from build123d import *

# Parameters (mm, degrees)
F0_W      = 30
F0_H      = 30
F1_DEPTH  = 20
F3_DEPTH  = 30.001
F7_W      = 5
F7_H      = 4
F8_DEPTH  = 3
F10_DEPTH = 1.5
F11_W     = 20
F11_H     = 12.5
F12_DEPTH = 9.9508743711
F13_W     = 30
F13_H     = 8
F14_DEPTH = 2
F15_R     = 1.25
F16_DEPTH = 5


with BuildPart() as f1:
    # F0 (on Front) → F1 (new body)
    with BuildSketch(Plane.XZ):
        with Locations((15, 15)):
            Rectangle(F0_W, F0_H)
    extrude(amount=F1_DEPTH)

    # F2 (on face) → F3 (cut, through all)
    with BuildSketch(Plane.XY.offset(30)):
        with BuildLine():
            Line((0, -20), (30, -20))
            ThreePointArc((30, -20), (15, -11.9498743711), (0, -20))
        make_face()
    extrude(amount=-F3_DEPTH, mode=Mode.SUBTRACT)

    # F7 (on offset) → F8 (cut)
    with BuildSketch(Plane.XZ.offset(12.9498743711)):
        with Locations((15, 15)):
            Rectangle(F7_W, F7_H)
    extrude(amount=-F8_DEPTH, mode=Mode.SUBTRACT)

    # F9 (on face) → F10 (cut)
    with BuildSketch(Plane.XY.offset(13)):
        with BuildLine():
            ThreePointArc((12.5, -12.1243309011), (15, -11.9498743711), (17.5, -12.1243309011))
            Line((17.5, -12.1243309011), (17.5, -9.9498743711))
            Line((17.5, -9.9498743711), (12.5, -9.9498743711))
            Line((12.5, -9.9498743711), (12.5, -12.1243309011))
        make_face()
    extrude(amount=-F10_DEPTH, mode=Mode.SUBTRACT)

    # F11 (on face) → F12 (cut, through all)
    with BuildSketch(Plane.XZ.offset(9.9498743711)):
        with Locations((15, 6.25)):
            Rectangle(F11_W, F11_H)
    extrude(amount=-F12_DEPTH, mode=Mode.SUBTRACT)

    # F13 (on face) → F14 (cut)
    with BuildSketch(Plane.XZ):
        with Locations((15, 15)):
            Rectangle(F13_W, F13_H)
    extrude(amount=F14_DEPTH, mode=Mode.SUBTRACT)

    # F15 (on face) → F16 (cut)
    with BuildSketch(Plane(origin=(0, 0, 12.5), x_dir=(1, 0, 0), z_dir=(0, 0, -1))):
        with Locations((18, 6.9498743711)):
            Circle(F15_R)
        with Locations((12, 6.9498743711)):
            Circle(F15_R)
    extrude(amount=-F16_DEPTH, mode=Mode.SUBTRACT)


solid = f1.part
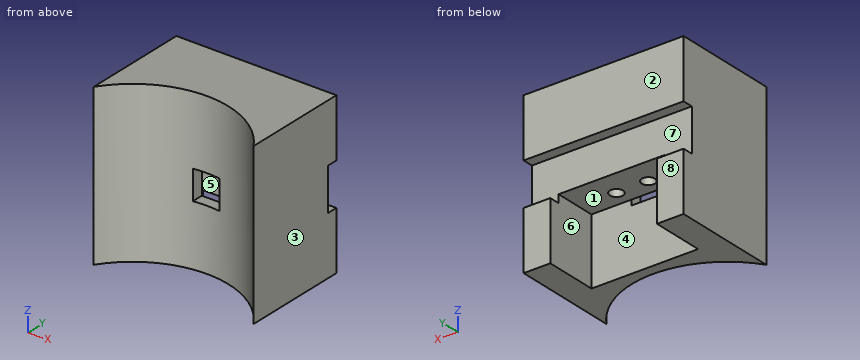
Source: CAD feature listing. Evaluate the final solid. Frame: model axes, mm. Face numbers are marked on the shaded views. A direction names the side the tool comes from. Round coordinates to 2 decimals unless told otherwise and drop trailing zeros. Loops run counter-clockwise (first coordinate to the right, second up) from the corner with the lowest first, then second, coordinate; pieces in that order, holes last.
Q1. First-contact query: P1, Ø6.5, axis at x = 15.5, y = -4, coming from the -Z side; P2, Ø6.5, axis at x = 16, z = 13.5, coming from the +Y side; P3, Ø1.1, axis at x = 16, y = -11, coming from the -Z side; P4, Ø1.3, axis at x = 16, z = 13.5, coming from the -Y side. Flat tips, straight axial feed; report the tip coordinate or a pass-through.
Q2. Access query for the marked faces 5, 6, 7 and 8. Directions: +Z, -Z, +X, -X, +Y, -Y. A direction counts if a zero-diameter tool reaches every point of the face in a straight line with its end or side. Return the directions, or none.
Q3. Section D-D, the plane y = -4.25. Return loops of the section in (x, z).
Q4. Section B-B, the plane z = 15.5. Return loops of the section in (x, y).
Q5. Section A-A, the plane y = -17.25. Return loops of the section in (x, z), plus the area to 3 significant figures.
Q6. Mould query, pull axis X, two halves, no side actions, for the marked faces 1, 2, 3 and 4. Classes: pulls with the +X half, pulls with the -X half, needs draft (parallel to the pull), parting line crosses it, or undercut.
Q7. Ray query, line 1 (X direction, y = -17, z = 4.75); line 2 (X direction, y = -14.5, z = 4.75); line 3 (Y direction, x = 15, z = 13.5). Return the intervals inside material, ascending.
Q8. Section C-C, the plane x = 14. Return loops of the section in (y, z).
Solutions:
1. P1: stops at z = 12.5
1. P2: stops at y = -2
1. P3: stops at z = 0
1. P4: stops at y = -9.95
2. face 5: -Y
2. face 6: -Z, +Y
2. face 7: +X, -X, +Y
2. face 8: +Z, -Z, +X, -X, +Y
3. outline: (0, 0) - (5, 0) - (5, 12.5) - (25, 12.5) - (25, 0) - (30, 0) - (30, 30) - (0, 30) - close
4. outline: (0, -20) arc R18 cw to (12.5, -12.12) - (12.5, -9.95) - (17.5, -9.95) - (17.5, -12.12) arc R18 cw to (30, -20) - (30, -2) - (0, -2) - close; hole circle Ø2.5 at (12, -6.95); hole circle Ø2.5 at (18, -6.95)
5. outline: (0, 0) - (2.24, 0) - (2.24, 30) - (0, 30) - close; (27.76, 0) - (30, 0) - (30, 30) - (27.76, 30) - close
5. area: 135 mm2
6. face 1: undercut
6. face 2: needs draft
6. face 3: pulls with the +X half
6. face 4: undercut
7. line 1: x = 0 to 2.5, 27.5 to 30
7. line 2: x = 0 to 5.76, 24.24 to 30
7. line 3: y = -9.95 to -2
8. outline: (-11.98, 0) - (-9.95, 0) - (-9.95, 11.5) - (-11.98, 11.5) - close; (-11.98, 17) - (-9.95, 17) - (-9.95, 12.5) - (-2, 12.5) - (-2, 19) - (0, 19) - (0, 30) - (-11.98, 30) - close
